Geometry: final body of the model. Coordinates: model frame, mm. A direction names the side the tool comes from. Give positions to 0.01 mm unless a question says otherwise; leave off trailing zeros. Write each loop counter-clockwise with the first axis right and the second up, starting at its lowest first coordinate (ties: lowest second). Pieces come first, ordered by that corner, then holes. Notation, with made-up numbers: M 18,47 L 33,47 A32 ccw 33,75 Z; hole C 22,37.25 d1. An arc over 180 degrees is marked long. Answer as a JSON object with one key per item and string values.
from build123d import *

# Parameters (mm, degrees)
F1_DEPTH = 15


with BuildPart() as f1:
    # F0 (on Right) → F1 (new body)
    with BuildSketch(Plane.YZ):
        with BuildLine():
            Line((-20, -20), (-10, -20))
            Line((-10, -20), (10, -20))
            Line((10, -20), (20, -20))
            Line((20, -20), (20, -15))
            ThreePointArc((20, -15), (18.535534, -11.464466), (15, -10))
            Line((15, -10), (10, -10))
            Line((10, -10), (10, 14.641016))
            Line((10, 14.641016), (-10, 20))
            Line((-10, 20), (-10, -10))
            Line((-10, -10), (-15, -10))
            ThreePointArc((-15, -10), (-18.535534, -11.464466), (-20, -15))
            Line((-20, -15), (-20, -20))
        make_face()
        Polygon((-4.211055, 13.992027), (4.314648, 11.707572), (2.968838, 6.684938), (-5.556865, 8.969393), align=None, mode=Mode.SUBTRACT)
    extrude(amount=F1_DEPTH)


solid = f1.part
1) Cut plane C-C on y = -3. Return loops of the section in (x, z), and give its area (3 significant figures).
Geometry check:
{"outline": "M 0,-20 L 15,-20 L 15,8.28 L 0,8.28 Z; M 0,13.67 L 15,13.67 L 15,18.12 L 0,18.12 Z", "area": "491 mm2"}
2) Pull-direction query (Z, two-part tool) for faces 1 (the flat face through (7.395, -0.008, 12.866)), 2 (the flat face through (7, 20, -18)), 3 (the cylindrical face through (7, -18, -11)); classes: pulls with the +Z half, pulls with the -Z half, needs draft (parallel to the pull), parting line crosses it, or undercut.
Geometry check:
{"face 1": "undercut", "face 2": "needs draft", "face 3": "pulls with the +Z half"}
3) Cut plane D-D on y = -12.5. Return loops of the section in (x, z), and give its area (3 significant figures).
Geometry check:
{"outline": "M 0,-20 L 15,-20 L 15,-10 L 0,-10 Z", "area": "150 mm2"}
4) Cut plane B-B on z = 10. Return loops of the section in (x, y), and give its area (3 significant figures).
Geometry check:
{"outline": "M 0,-10 L 15,-10 L 15,-5.28 L 0,-5.28 Z; M 0,3.86 L 15,3.86 L 15,10 L 0,10 Z", "area": "163 mm2"}
5) Cut plane A-A on x = 7.75. Return loops of the section in (y, z), and give its area (3 significant figures).
Geometry check:
{"outline": "M -20,-20 L 20,-20 L 20,-15 A5 ccw 15,-10 L 10,-10 L 10,14.64 L -10,20 L -10,-10 L -15,-10 A5 ccw -20,-15 Z; hole M -5.56,8.97 L 2.97,6.68 L 4.31,11.71 L -4.21,13.99 Z", "area": "890 mm2"}
6) Line query: line 1 (Y direction, x = 9, z = -0.5); line 2 (Y direction, x = 2.5, z = 11.5); line 3 (Z direction, x = 14, y = 0). Output: solid intervals per line, ascending. Write a range as from..to.
Geometry check:
{"line 1": "y = -10..10", "line 2": "y = -10..-4.88, 4.26..10", "line 3": "z = -20..7.48, 12.86..17.32"}
7) Set-up query: faces 4 (the flat face through (15, 0, -4)), 5 (the flat face through (7.395, -4.893, 11.446)), 6 (the flat face through (7, 0, -20)), 7 (the flat face through (7, -12, -10)), 8 (the flat face through (7, 13, -10)). Return all of +Z, -Z, +X, -X, +Y, -Y with unobstructed straight access to the full face (end or side cutting, diameter ignored); none if empty.
Geometry check:
{"face 4": "+Z, -Z, +X, +Y, -Y", "face 5": "+X, -X", "face 6": "-Z, +X, -X, +Y, -Y", "face 7": "+Z, +X, -X, -Y", "face 8": "+Z, +X, -X, +Y"}
8) Contact query for flat-ended pins moving along their axis: P1, Ø3, axis at x = 5, y = -4.5, coming from the +Z side; P2, Ø7.5, axis at x = 7, z = -0.5, coming from the +Y side; P3, Ø4, axis at x = 8.5, y = -9.5, coming from the +Z side. Output: stop coordinate, or through.
Geometry check:
{"P1": "stops at z = 18.93", "P2": "stops at y = 10", "P3": "stops at z = 20"}
